The model under review builds one solid part; all positions refer to its coordinate system, in mm. Coordinates: 2 decimals unless noted, no trailing zeros. Order: outer loops, then holes, each group sorted by start corner. A loop starts at its lowest first (then second) coordinate and runs counter-clockwise, first axis right, second up. Notation, with made-up numbers: (66.25, -6.5) -> (112.25, -6.5) arc R24 ccw to (112.25, 30.5) -> close; hole circle Ø5 at (31.5, 56.25). An arc over 180 degrees is marked (long way). Put each result on its own line as item: value.
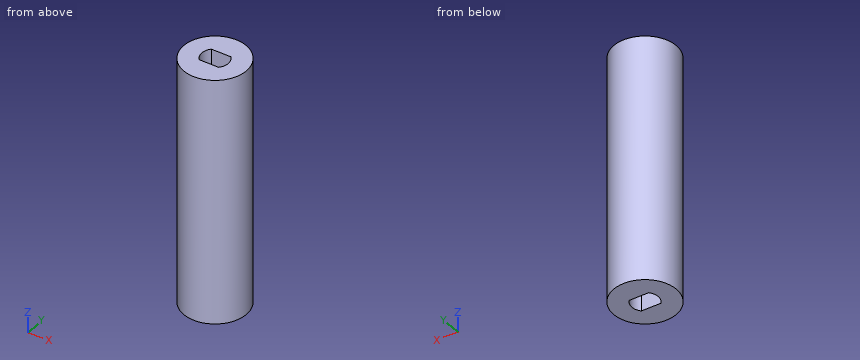
Autodesk Inventor part; units mm, degrees
ref_plane "YZ Plane" through (0, 0, 0) normal (1, 0, 0) x (0, 1, 0)
ref_plane "XZ Plane" through (0, 0, 0) normal (0, 1, 0) x (-1, 0, 0)
ref_plane "XY Plane" through (0, 0, 0) normal (0, 0, 1) x (1, 0, 0)
sketch "Boceto1" plane through (2.1662, 2, 0) normal (0, 0, -1) x (-1, 0, 0)
  line L0 (4.3355, -4) -> (-0.0031, -4)
  line L1 (4.3355, 0) -> (-0.0031, 0)
  arc A0 (4.3355, -4) -> (4.3355, 0) centre (2.1662, -2) ccw
  arc A1 (-0.0031, 0) -> (-0.0031, -4) centre (2.1662, -2) ccw
  circle A2 centre (2.1662, -2) radius 6.9999
extrude "Extrusión1" add sketch "Boceto1" along normal blind 55
properties part number "Rodamiento_Motor_X2"
Item 1: Consider section D-D on y = -3.5. Write out the cut boundary in (x, z), and give its area (3 significant figures).
Answers below:
outline: (-6.06, -55) -> (6.06, -55) -> (6.06, 0) -> (-6.06, 0) -> close
area: 667 mm^2
Item 2: Consider section C-C on z = -28. Write out the cut boundary in (x, y), and give its area (3 significant figures).
Answers below:
outline: circle Ø14 at (0, 0); hole (-2.17, -2) -> (2.17, -2) arc R2.95 ccw to (2.17, 2) -> (-2.17, 2) arc R2.95 ccw to start
area: 132 mm^2
Item 3: For line 1 (Y direction, x = -1.25, z = -11); line 2 (X direction, y = -1, z = -26); line 3 (Y direction, x = 2, z = -3.5), list the stretches that pass through material, from the lowest coordinate up. Write a range as from..to.
Answers below:
line 1: -6.89..-2, 2..6.89
line 2: -6.93..-2.78, 2.78..6.93
line 3: -6.71..-2, 2..6.71
Item 4: Consider section B-B on y = -0.5. Write out the cut boundary in (x, z), and give its area (3 significant figures).
Answers below:
outline: (-6.98, -55) -> (-2.91, -55) -> (-2.91, 0) -> (-6.98, 0) -> close; (2.91, -55) -> (6.98, -55) -> (6.98, 0) -> (2.91, 0) -> close
area: 448 mm^2
Item 5: For pin 1 Ø4 at (y, z) = (2.5, -36.5) entering from +X, flat-tipped, find the tip position at first contact; note if it passes through.
Answers below:
pin 1: x = 6.98
Item 6: Consider section A-A on x = 0. Write out the cut boundary in (y, z), and give its area (3 significant figures).
Answers below:
outline: (-7, -55) -> (-2, -55) -> (-2, 0) -> (-7, 0) -> close; (2, -55) -> (7, -55) -> (7, 0) -> (2, 0) -> close
area: 550 mm^2
